Read the model definition and answer for the solid it produces. Units are mm, in the model's axes. Give positions to 0.01 mm unless a question says otherwise; leave off trailing zeros. Write each loop counter-clockwise with the first axis right and the second up, starting at its lowest first coordinate (ties: lowest second). Pieces come first, ordered by that corner, then holes. Notation, with made-up numbers: (28.25, 19.5) - (34.25, 19.5) arc R17 cw to (34.25, 47.5) - close; hole circle Ø6 at (84.25, 61). An arc over 180 degrees is marked (long way). Answer as CSV lines item,"result".
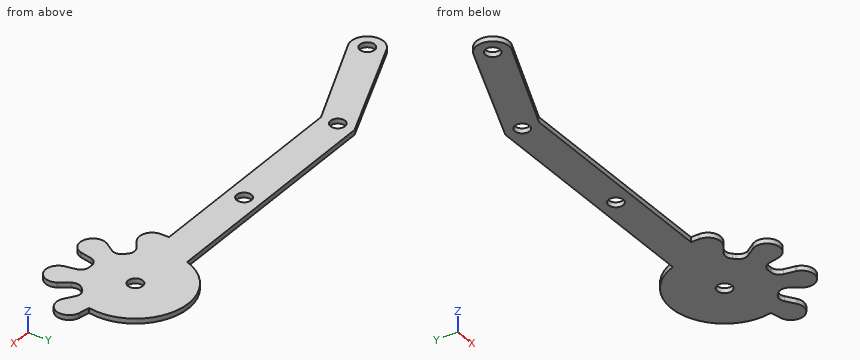
```python
from build123d import *

# Parameters (mm, degrees)
MODEL_R                 = 1.5
SALIENTE_EXTRUIR1_DEPTH = 1


with BuildPart() as part:
    # Model → Saliente-Extruir1 (new body)
    with BuildSketch(Plane.XY):
        with BuildLine():
            Line((6.261217919, 18.769360839), (-14.739513879, 9.794996238))
            ThreePointArc((-14.739513879, 9.794996238), (-18.828558612, 11.883464999), (-16.872209477, 16.037341099))
            Line((-16.872209477, 16.037341099), (6.261217919, 25.600360839))
            Line((6.261217919, 25.600360839), (33.761217919, 25.600360839))
            Line((33.761217919, 25.600360839), (55.398917602, 25.600360839))
            ThreePointArc((55.398917602, 25.600360839), (68.422679159, 32.642144419), (76.271846628, 20.088433767))
            Line((76.271846628, 20.088433767), (78.346726924, 19.678483017))
            ThreePointArc((78.346726924, 19.678483017), (78.464143806, 19.652436824), (78.580224549, 19.620966371))
            Line((78.580224549, 19.620966371), (78.611928195, 19.611354587))
            ThreePointArc((78.611928195, 19.611354587), (80.237076178, 16.147342665), (76.638496698, 14.847069503))
            Line((76.638496698, 14.847069503), (76.609282278, 14.862690809))
            ThreePointArc((76.609282278, 14.862690809), (76.504947826, 14.922519319), (76.403504113, 14.987128153))
            Line((76.403504113, 14.987128153), (74.575103444, 16.212224841))
            ThreePointArc((74.575103444, 16.212224841), (73.415610314, 16.492916463), (72.35097411, 15.954621135))
            Line((72.35097411, 15.954621135), (71.891457622, 15.495104647))
            ThreePointArc((71.891457622, 15.495104647), (71.353162294, 14.430468442), (71.633853917, 13.270975311))
            Line((71.633853917, 13.270975311), (72.858950606, 11.442574643))
            ThreePointArc((72.858950606, 11.442574643), (72.92355944, 11.34113093), (72.98338795, 11.236796479))
            Line((72.98338795, 11.236796479), (72.999009256, 11.207582059))
            ThreePointArc((72.999009256, 11.207582059), (71.698736047, 7.609002556), (68.234724141, 9.234150662))
            Line((68.234724141, 9.234150662), (68.225112387, 9.265854208))
            ThreePointArc((68.225112387, 9.265854208), (68.193641935, 9.381934951), (68.167595742, 9.499351833))
            Line((68.167595742, 9.499351833), (67.740995408, 11.65850052))
            ThreePointArc((67.740995408, 11.65850052), (67.119588901, 12.676864925), (65.986145145, 13.049044127))
            Line((65.986145145, 13.049044127), (65.336290696, 13.049044127))
            ThreePointArc((65.336290696, 13.049044127), (64.20284694, 12.676864925), (63.581440434, 11.658500522))
            Line((63.581440434, 11.658500522), (63.154840098, 9.499351834))
            ThreePointArc((63.154840098, 9.499351834), (63.128793905, 9.381934952), (63.097323452, 9.265854209))
            Line((63.097323452, 9.265854209), (63.087711668, 9.234150563))
            ThreePointArc((63.087711668, 9.234150563), (59.623699794, 7.609002564), (58.323426536, 11.20758197))
            Line((58.323426536, 11.20758197), (58.33904789, 11.23679648))
            ThreePointArc((58.33904789, 11.23679648), (58.3988764, 11.341130932), (58.463485233, 11.442574645))
            Line((58.463485233, 11.442574645), (59.688581925, 13.270975312))
            ThreePointArc((59.688581925, 13.270975312), (59.969273546, 14.430468443), (59.430978219, 15.495104647))
            Line((59.430978219, 15.495104647), (58.971461731, 15.954621135))
            ThreePointArc((58.971461731, 15.954621135), (57.906825526, 16.492916463), (56.747332395, 16.21222484))
            Line((56.747332395, 16.21222484), (54.918931727, 14.987128151))
            ThreePointArc((54.918931727, 14.987128151), (54.817488014, 14.922519317), (54.713153563, 14.862690807))
            Line((54.713153563, 14.862690807), (54.683939143, 14.847069501))
            ThreePointArc((54.683939143, 14.847069501), (52.139490235, 14.921450429), (50.888257342, 17.138242934))
            Line((50.888257342, 17.138242934), (50.888257342, 18.769360839))
            Line((50.888257342, 18.769360839), (6.261217919, 18.769360839))
        make_face()
        with Locations((65.661217919, 22.184860839)):
            Circle(MODEL_R, mode=Mode.SUBTRACT)
        with Locations((33.761217919, 22.184860839)):
            Circle(MODEL_R, mode=Mode.SUBTRACT)
        with Locations((6.261217919, 22.184860839)):
            Circle(MODEL_R, mode=Mode.SUBTRACT)
        with Locations((-15.705782081, 12.950360839)):
            Circle(MODEL_R, mode=Mode.SUBTRACT)
    extrude(amount=SALIENTE_EXTRUIR1_DEPTH)


solid = part.part
```
(1) A cutting plane is placed at C-C (y = 28.5). Write down the section's boundary in (x, z).
Worked out:
outline,"(56.88, 0) - (74.44, 0) - (74.44, 1) - (56.88, 1) - close"
(2) A cutting plane is placed at B-B (z = 0.4). Count the separate pieces of the cut face and the enclosed holes in it, and give its area (3 significant figures).
Worked out:
separate pieces,"1"
enclosed holes,"4"
area,"912 mm^2"
(3) A cutting plane is placed at A-A (x = 28). Write down the section's boundary in (y, z).
Worked out:
outline,"(18.77, 0) - (25.6, 0) - (25.6, 1) - (18.77, 1) - close"
(4) Find the intervals of material crossed by L1, parallel to X at y = 13.75, z = 0.3; L2, parallel to X at y = 22.25, z = 0.5; L3, parallel to X at y = 23.25, z = 0.9, in increasing order.
Worked out:
L1,"x = -18.91 to -16.97, -14.44 to -5.48, 59.91 to 71.41"
L2,"x = -1.84 to 4.76, 7.76 to 32.26, 35.26 to 64.16, 67.16 to 76.48"
L3,"x = 0.58 to 5.21, 7.32 to 32.71, 34.82 to 64.61, 66.72 to 76.42"
